Design review of the part shown in the three views and the two pictorial views. Dimensions are in mm from the part's minimum x, y and z. Coordinates: 2 decimals unless noted, no trailing zeros. Loops run counter-clockwise (first coordinate to the right, second up) from the corner with the lowest first, then second, coordinate; pieces in that order, holes last. Notation, with made-up numbers: (6, 33.25) -> (14, 33.25) arc R19 ccw to (14, 49.25) -> close; hole circle Ø11 at (12.25, 51). An arc over 180 degrees is marked (long way). Answer in a Markdown table with one row per item.
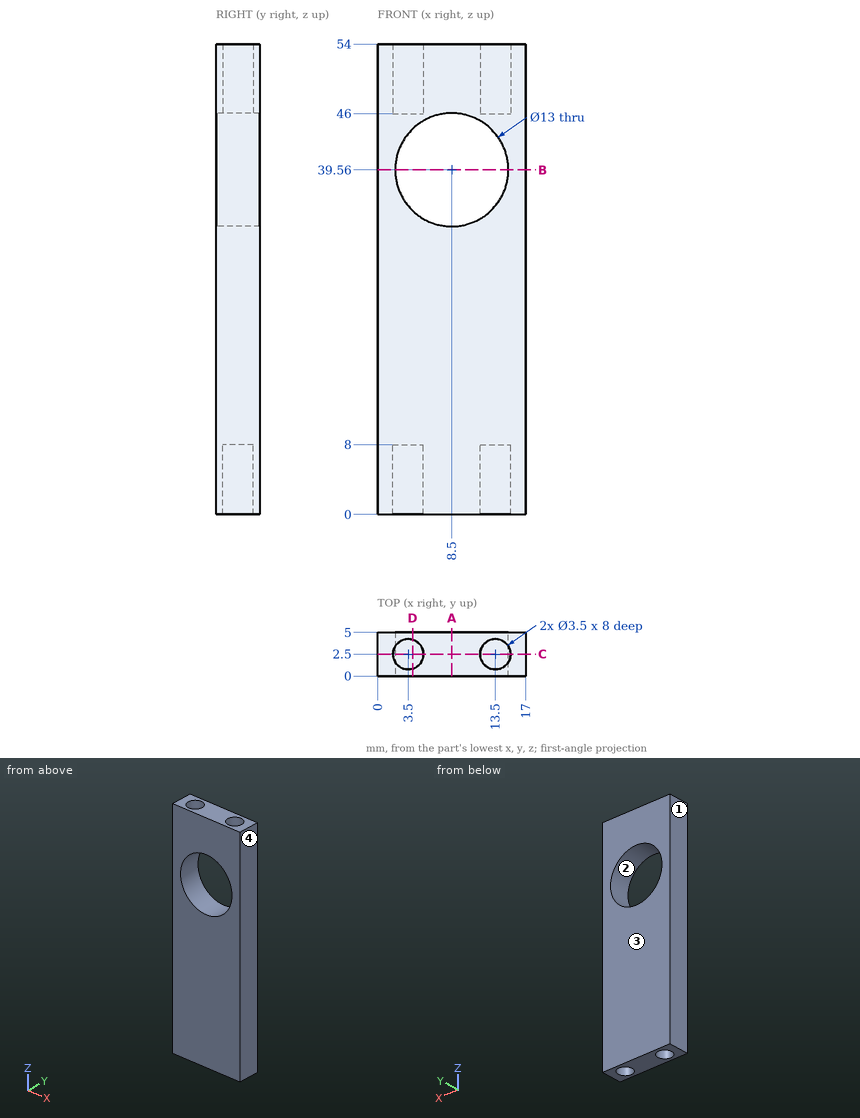
Item 1: Take a section at D-D, the plane x = 4. State the section outline as (y, z) points, and give its area (3 significant figures).
Worked answers:
| item | result |
|---|---|
| outline | (0, 0) -> (0.82, 0) -> (0.82, 8) -> (4.18, 8) -> (4.18, 0) -> (5, 0) -> (5, 34.87) -> (0, 34.87) -> close; (0, 44.25) -> (5, 44.25) -> (5, 54) -> (4.18, 54) -> (4.18, 46) -> (0.82, 46) -> (0.82, 54) -> (0, 54) -> close |
| area | 169 mm² |
Item 2: Take a section at C-C, the plane y = 2.5. State the section outline as (x, z) points.
Worked answers:
| item | result |
|---|---|
| outline | (0, 0) -> (1.75, 0) -> (1.75, 8) -> (5.25, 8) -> (5.25, 0) -> (11.75, 0) -> (11.75, 8) -> (15.25, 8) -> (15.25, 0) -> (17, 0) -> (17, 54) -> (15.25, 54) -> (15.25, 46) -> (11.75, 46) -> (11.75, 54) -> (5.25, 54) -> (5.25, 46) -> (1.75, 46) -> (1.75, 54) -> (0, 54) -> close; hole circle Ø13 at (8.5, 39.56) |
Item 3: Take a section at A-A, the plane x = 8.5. State the section outline as (y, z) points, and give its area (3 significant figures).
Worked answers:
| item | result |
|---|---|
| outline | (0, 0) -> (5, 0) -> (5, 33.06) -> (0, 33.06) -> close; (0, 46.06) -> (5, 46.06) -> (5, 54) -> (0, 54) -> close |
| area | 205 mm² |
Item 4: Take a section at B-B, the plane z = 39.56. State the section outline as (x, y) points, and give its area (3 significant figures).
Worked answers:
| item | result |
|---|---|
| outline | (0, 0) -> (2, 0) -> (2, 5) -> (0, 5) -> close; (15, 0) -> (17, 0) -> (17, 5) -> (15, 5) -> close |
| area | 20.0 mm² |
Item 5: The part is to be moulded in two halves that separate along X. For the marked faces 1, 2, 3 and 4, say which applies: +X half, -X half, draft (parallel to the pull), parting line (faces both ways), or undercut.
Worked answers:
| item | result |
|---|---|
| face 1 | -X half |
| face 2 | undercut |
| face 3 | draft |
| face 4 | +X half |
Item 6: For L1, parallel to X at y = 2.5, z = 48.5; L2, parallel to Y at x = 3.5, z = 49.5; L3, parallel to Z at x = 8.5, y = 1.55, list the stretches that pass through material, from the lowest coordinate up.
Worked answers:
| item | result |
|---|---|
| L1 | 0 to 1.75, 5.25 to 11.75, 15.25 to 17 |
| L2 | 0 to 0.75, 4.25 to 5 |
| L3 | 0 to 33.06, 46.06 to 54 |
Item 7: Insertion check: pin 1 (3 mm diameter, centred on x = 3.5, y = 2.5, fed in from +Z); pin 2 (3 mm diameter, centred on x = 5, z = 39.5, fed in from +Y). Each pin has a flat end and moves straight along its axis. Give the tip position at first contact, or say it passes through.
Worked answers:
| item | result |
|---|---|
| pin 1 | z = 46 |
| pin 2 | through |
